```python
from build123d import *

# Parameters (mm, degrees)
SKETCH1_W           = 101.6
SKETCH1_H           = 76.2
BOSS_EXTRUDE1_DEPTH = 25.4
SKETCH2_R           = 2.794
CUT_EXTRUDE1_DEPTH  = 10.16
SHELL1_DEPTH        = 22.86
SHELL1_START        = 12.7
SHELL1_2_DEPTH      = 10.16


# Read off the part's stored shape, not the designer's step: Shell1
with BuildPart() as part:
    # Sketch1 → Boss-Extrude1 (new body)
    with BuildSketch(Plane.XY):
        Rectangle(SKETCH1_W, SKETCH1_H)
    extrude(amount=BOSS_EXTRUDE1_DEPTH)

    # Sketch2 → Cut-Extrude1 (cut)
    with BuildSketch(Plane(origin=(0, 0, 0), x_dir=(-1, 0, 0), z_dir=(0, 0, -1))):
        with Locations((45.72, -33.02)):
            Circle(SKETCH2_R)
        with Locations((-45.72, -33.02)):
            Circle(SKETCH2_R)
        with Locations((-45.72, 33.02)):
            Circle(SKETCH2_R)
        with Locations((45.72, 33.02)):
            Circle(SKETCH2_R)
    extrude(amount=-CUT_EXTRUDE1_DEPTH, mode=Mode.SUBTRACT)

    # Shell1 outline → Shell1 (cut)
    with BuildSketch(Plane.XY):
        with BuildLine():
            Line((41.029588931, 35.56), (-41.029588931, 35.56))
            ThreePointArc((-41.029588931, 35.56), (-41.948292429, 29.248292429), (-48.26, 28.329588931))
            Line((-48.26, 28.329588931), (-48.26, -28.329588931))
            ThreePointArc((-48.26, -28.329588931), (-41.948292429, -29.248292429), (-41.029588931, -35.56))
            Line((-41.029588931, -35.56), (41.029588931, -35.56))
            ThreePointArc((41.029588931, -35.56), (41.948292429, -29.248292429), (48.26, -28.329588931))
            Line((48.26, -28.329588931), (48.26, 28.329588931))
            ThreePointArc((48.26, 28.329588931), (41.948292429, 29.248292429), (41.029588931, 35.56))
        make_face()
    extrude(amount=SHELL1_DEPTH, mode=Mode.SUBTRACT)

    # Shell1 2 outline → Shell1 2 (cut)
    with BuildSketch(Plane.XY.offset(SHELL1_START)):
        with BuildLine():
            Line((-41.029588931, 35.56), (-48.26, 35.56))
            Line((-48.26, 35.56), (-48.26, 28.329588931))
            ThreePointArc((-48.26, 28.329588931), (-41.948292429, 29.248292429), (-41.029588931, 35.56))
        make_face()
        with BuildLine():
            Line((48.26, 35.56), (41.029588931, 35.56))
            ThreePointArc((41.029588931, 35.56), (41.948292429, 29.248292429), (48.26, 28.329588931))
            Line((48.26, 28.329588931), (48.26, 35.56))
        make_face()
        with BuildLine():
            ThreePointArc((-41.029588931, -35.56), (-41.948292429, -29.248292429), (-48.26, -28.329588931))
            Line((-48.26, -28.329588931), (-48.26, -35.56))
            Line((-48.26, -35.56), (-41.029588931, -35.56))
        make_face()
        with BuildLine():
            Line((48.26, -35.56), (48.26, -28.329588931))
            ThreePointArc((48.26, -28.329588931), (41.948292429, -29.248292429), (41.029588931, -35.56))
            Line((41.029588931, -35.56), (48.26, -35.56))
        make_face()
    extrude(amount=SHELL1_2_DEPTH, mode=Mode.SUBTRACT)


solid = part.part
```
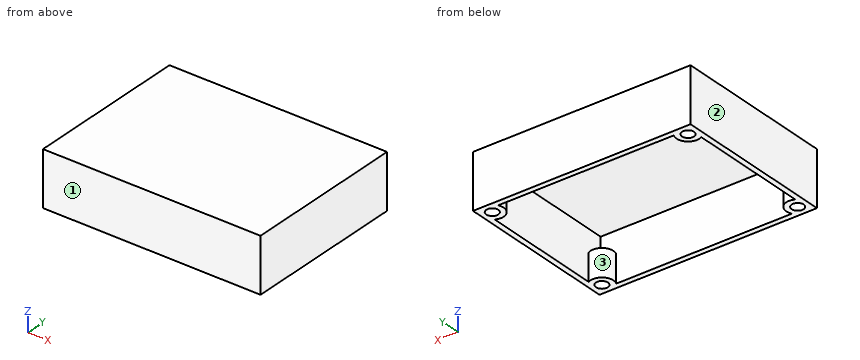
Design review of the part built by this model. Coordinates are the model's own, in mm. Face numbers are marked on the shaded views. Give positions to 0.01 mm unless a question says otherwise; leave off trailing zeros. Write each loop counter-clockwise with the first axis right and the second up, starting at its lowest first coordinate (ties: lowest second). Pieces come first, ordered by that corner, then holes. Notation, with made-up numbers: (61.5, 84.5) - (101.5, 84.5) arc R13 cw to (101.5, 98.5) - close; hole circle Ø5 at (84.25, -11.5). An arc over 180 degrees is marked (long way). Return JSON: item names as keys, results as strings. Group by question number.
(1) Mouldability with a two-part tool opening along Y and no side actions: class the marked faces 1, 2 and 3 as +Y half, -Y half, draft (parallel to the pull), parting line (faces both ways), or undercut.
(2) Insertion check: pin 1 (8 mm diameter, centred on x = 31.5, y = 18.5, fed in from -Z); pin 2 (5 mm diameter, centred on x = -45.72, y = -33.02, fed in from -Z). Each pin has a flat end and moves straight along its axis. Give the tip position at first contact, or say it passes through.
(3) We need section D-D, the plane x = 7.5. Give the boundary of the cut face in (y, z).
(4) To check wall thickness, follow probe 1 along Y at (x, z) = (-45.72, 4.5); probe 2 along Y at (x, z) = (8, 4); probe 3 along X at (y, z) = (0.5, 20). State the ranges of each line that lie inside material, in increasing order.
(5) We need section A-A, the plane x = 45.72. Give the boundary of the cut face in (y, z).
(6) We need section B-B, the plane y = -13. Give the boundary of the cut face in (x, z).
(7) We need section C-C, the plane z = 5.5. Give the boundary of the cut face in (x, y), then the cut area to 3 significant figures.
Reported:
{
 "1": {"face 1": "-Y half", "face 2": "draft", "face 3": "undercut"},
 "2": {"pin 1": "stops at z = 22.86", "pin 2": "stops at z = 10.16"},
 "3": {"outline": "(-38.1, 0) - (-35.56, 0) - (-35.56, 22.86) - (35.56, 22.86) - (35.56, 0) - (38.1, 0) - (38.1, 25.4) - (-38.1, 25.4) - close"},
 "4": {"probe 1": "y = -38.1 to -35.81, -30.23 to -27.69, 27.69 to 30.23, 35.81 to 38.1", "probe 2": "y = -38.1 to -35.56, 35.56 to 38.1", "probe 3": "x = -50.8 to -48.26, 48.26 to 50.8"},
 "5": {"outline": "(-38.1, 0) - (-35.81, 0) - (-35.81, 10.16) - (-30.23, 10.16) - (-30.23, 0) - (-27.69, 0) - (-27.69, 12.7) - (-35.56, 12.7) - (-35.56, 22.86) - (35.56, 22.86) - (35.56, 12.7) - (27.69, 12.7) - (27.69, 0) - (30.23, 0) - (30.23, 10.16) - (35.81, 10.16) - (35.81, 0) - (38.1, 0) - (38.1, 25.4) - (-38.1, 25.4) - close"},
 "6": {"outline": "(-50.8, 0) - (-48.26, 0) - (-48.26, 22.86) - (48.26, 22.86) - (48.26, 0) - (50.8, 0) - (50.8, 25.4) - (-50.8, 25.4) - close"},
 "7": {"outline": "(-50.8, -38.1) - (50.8, -38.1) - (50.8, 38.1) - (-50.8, 38.1) - close; hole circle Ø5.59 at (-45.72, -33.02); hole circle Ø5.59 at (-45.72, 33.02); hole (-48.26, -28.33) arc R5.33 cw to (-41.03, -35.56) - (41.03, -35.56) arc R5.33 cw to (48.26, -28.33) - (48.26, 28.33) arc R5.33 cw to (41.03, 35.56) - (-41.03, 35.56) arc R5.33 cw to (-48.26, 28.33) - close; hole circle Ø5.59 at (45.72, -33.02); hole circle Ø5.59 at (45.72, 33.02)", "area": "999 mm2"}
}
